```python
from build123d import *

# Parameters (mm, degrees)
F0_R     = 2.25
F0_R_2   = 1.5
F0_R_3   = 1.3
F1_DEPTH = 0.5
F2_DEPTH = 5
F3_R     = 1.55
F4_DEPTH = 0.5
F5_R     = 0.2


with BuildPart() as f1:
    # F0 (on Top) → F1 (new body)
    with BuildSketch(Plane.XY):
        Circle(F0_R)
        Circle(F0_R_2, mode=Mode.SUBTRACT)
        Circle(F0_R_2)
        Circle(F0_R_3, mode=Mode.SUBTRACT)
        Circle(F0_R_3)
    extrude(amount=F1_DEPTH)

    # F0 (on Top) → F2 (join)
    with BuildSketch(Plane.XY):
        Circle(F0_R_3)
    extrude(amount=F2_DEPTH)

    # F3 (on face) → F4 (join)
    with BuildSketch(Plane.XY.offset(5)):
        Circle(F3_R)
    extrude(amount=-F4_DEPTH)

    # F5
    f5_edges = [f1.edges().sort_by_distance(p)[0] for p in [
        (-1.55, 0, 4.5),
        (-1.55, 0, 5),
    ]]
    fillet(f5_edges, radius=F5_R)


solid = f1.part
```
Part model, mm, in its own coordinate system. Coordinates: 2 decimals unless noted, no trailing zeros. Write each loop counter-clockwise with the first axis right and the second up, starting at its lowest first coordinate (ties: lowest second). Pieces come first, ordered by that corner, then holes.
Item 1: Probe line 1 (Z direction, x = -1, y = -0.9); line 2 (Z direction, x = 1.8, y = 1.1); line 3 (X direction, y = 0.05, z = 1.85). List the from-to ranges inside material, lowest first.
Item 2: Mould opens along Z. For faces 1 (the face through (0, 0, 5)), 2 (the face through (0, 0, 0)), 3 (the face through (-0.17, 1.29, 2.47)), 4 (the face through (0, -1.5, 0.5)) say: released by +Z, released by -Z, zero draft, split by the parting line, or undercut.
Item 3: Slice it at A-A (y = 0). Write the cut outline in (x, z).
Item 4: Slice it at C-C (z = 1.85). Write the cut outline in (x, y), and give its area (3 significant figures).
Item 5: Pin check, flat tips, straight feed: pin 1 (1 mm diameter, centred on x = -2, y = -2, fed in from +Z); pin 2 (1 mm diameter, centred on y = 0, z = 1.5, fed in from -X); pin 3 (1 mm diameter, centred on y = -1.5, z = 3, fed in from +X). Stop position of each tip, or through.
Item 6: Slice it at D-D (x = -1.7). Write the cut outline in (y, z).
Results found:
1. line 1: z = 0 to 0.5, 4.5 to 5
1. line 2: z = 0 to 0.5
1. line 3: x = -1.3 to 1.3
2. face 1: released by +Z
2. face 2: released by -Z
2. face 3: undercut
2. face 4: undercut
3. outline: (-2.25, 0) - (2.25, 0) - (2.25, 0.5) - (1.3, 0.5) - (1.3, 4.5) - (1.35, 4.5) arc R0.2 ccw to (1.55, 4.7) - (1.55, 4.8) arc R0.2 ccw to (1.35, 5) - (-1.35, 5) arc R0.2 ccw to (-1.55, 4.8) - (-1.55, 4.7) arc R0.2 ccw to (-1.35, 4.5) - (-1.3, 4.5) - (-1.3, 0.5) - (-2.25, 0.5) - close
4. outline: circle Ø2.6 at (0, 0)
4. area: 5.31 mm2
5. pin 1: passes through
5. pin 2: stops at x = -1.3
5. pin 3: stops at x = 0.83
6. outline: (-1.47, 0) - (1.47, 0) - (1.47, 0.5) - (-1.47, 0.5) - close
